```python
from build123d import *

# Parameters (mm, degrees)
BOSS_EXTRUDE1_DEPTH = 2
BOSS_EXTRUDE2_DEPTH = 0.9
SKETCH3_R           = 0.75
CUT_EXTRUDE1_DEPTH  = 0.9
SKETCH4_R           = 0.65
SKETCH4_R_2         = 1.5
CUT_EXTRUDE2_DEPTH  = 0.1
BOSS_EXTRUDE3_DEPTH = 1
SKETCH6_R           = 0.65
BOSS_EXTRUDE4_DEPTH = 5


with BuildPart() as part:
    # Sketch1 → Boss-Extrude1 (new body)
    with BuildSketch(Plane.XY):
        with BuildLine():
            Line((-7.95, 2.1), (7.95, 2.1))
            ThreePointArc((7.95, 2.1), (10.05, 0), (7.95, -2.1))
            Line((7.95, -2.1), (-7.95, -2.1))
            ThreePointArc((-7.95, -2.1), (-10.05, 0), (-7.95, 2.1))
        make_face()
    extrude(amount=BOSS_EXTRUDE1_DEPTH)

    # Sketch2 → Boss-Extrude2 (add)
    with BuildSketch(Plane.XY.offset(2)):
        with BuildLine():
            Line((-10.84, 2.1), (10.84, 2.1))
            ThreePointArc((10.84, 2.1), (12.94, 0), (10.84, -2.1))
            Line((10.84, -2.1), (-10.84, -2.1))
            ThreePointArc((-10.84, -2.1), (-12.94, 0), (-10.84, 2.1))
        make_face()
    extrude(amount=BOSS_EXTRUDE2_DEPTH)

    # Sketch3 → Cut-Extrude1 (cut)
    with BuildSketch(Plane(origin=(0, 0, 2), x_dir=(-1, 0, 0), z_dir=(0, 0, -1))):
        with Locations((-11.49, 0)):
            Circle(SKETCH3_R)
        with Locations((11.49, 0)):
            Circle(SKETCH3_R)
    extrude(amount=-CUT_EXTRUDE1_DEPTH, mode=Mode.SUBTRACT)

    # Sketch4 → Cut-Extrude2 (cut)
    with BuildSketch(Plane(origin=(0, 0, 0), x_dir=(-1, 0, 0), z_dir=(0, 0, -1))):
        Circle(SKETCH4_R)
        with Locations((2.54, 0)):
            Circle(SKETCH4_R)
        with Locations((5.08, 0)):
            Circle(SKETCH4_R)
        with Locations((-2.54, 0)):
            Circle(SKETCH4_R)
        with Locations((-5.08, 0)):
            Circle(SKETCH4_R)
        with Locations((-8, 0)):
            Circle(SKETCH4_R_2)
        with Locations((8, 0)):
            Circle(SKETCH4_R_2)
    extrude(amount=-CUT_EXTRUDE2_DEPTH, mode=Mode.SUBTRACT)

    # Sketch5 → Boss-Extrude3 (add)
    with BuildSketch(Plane.XY.offset(2.9)):
        with BuildLine():
            Line((7.95, 2.1), (-7.95, 2.1))
            ThreePointArc((-7.95, 2.1), (-10.05, 0), (-7.95, -2.1))
            Line((-7.95, -2.1), (7.95, -2.1))
            ThreePointArc((7.95, -2.1), (10.05, 0), (7.95, 2.1))
        make_face()
    extrude(amount=BOSS_EXTRUDE3_DEPTH)

    # Sketch6 → Boss-Extrude4 (add)
    with BuildSketch(Plane.XY.offset(3.9)):
        with Locations(Location((-5.08, 0, 0), (0, 0, 180))):
            Circle(SKETCH6_R)
        with Locations(Location((-2.54, 0, 0), (0, 0, 180))):
            Circle(SKETCH6_R)
        with Locations(Location((0, 0, 0), (0, 0, 180))):
            Circle(SKETCH6_R)
        with Locations(Location((2.54, 0, 0), (0, 0, 180))):
            Circle(SKETCH6_R)
        with Locations(Location((5.08, 0, 0), (0, 0, 180))):
            Circle(SKETCH6_R)
    extrude(amount=BOSS_EXTRUDE4_DEPTH)


solid = part.part
```
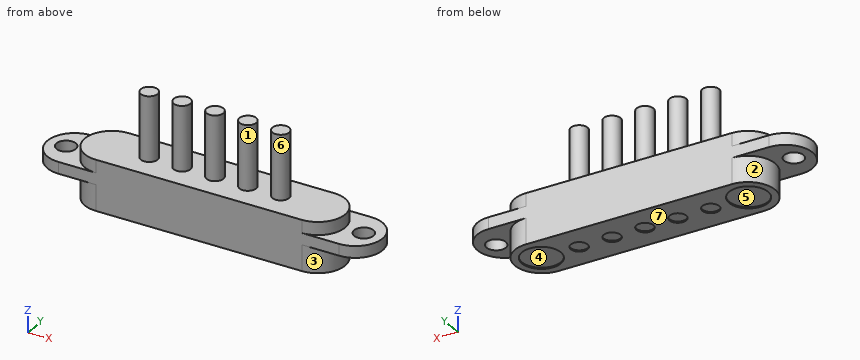
Could you check a few things on this model? Use its own coordinates, in mm. Face numbers are marked on the shaded views. A direction names the side the tool comes from. Give positions to 0.01 mm unless a question says otherwise; leave off trailing zeros. Order: outer loops, then holes, each group sorted by start corner. A loop starts at its lowest first (then second) coordinate and runs counter-clockwise, first axis right, second up.
Q1. Suppose I cut it at A-A, the plane z = 4.5. Write out the boundary of the cut face in (x, y).
Q2. If I drill on line 1 along Y through (x, z) = (8, 0.05); line 2 along Y through (x, z) = (-2.54, 0.05); line 3 along X through (y, z) = (-0.5, 2.75), over which ranges is the centre line in solid material (lowest first)?
Q3. I'm going to push flat-ended pins straight in: P1, Ø1.3, axis at x = -11, y = 0.5, coming from the +Z side; P2, Ø0.8, axis at x = -2.54, y = 0, coming from the -Z side; P3, Ø1.5, axis at y = 1.5, z = 4.5, coming from the +X side. Where does each tip first touch, or does it pass through?
Q4. Suppose I cut it at D-D, the plane y = -1.05. Write out the boundary of the cut face in (x, z).
Q5. Suppose I cut it at C-C, the plane x = -11.49. Write out the boundary of the cut face in (y, z).
Q6. We'd pull the mould along Y, two halves only. Please class the marked faces 5, 6 and 7: +Y half, -Y half, draft (parallel to the pull), parting line (faces both ways), or undercut.
Q7. Suppose I cut it at B-B, the plane x = 0. Write out the boundary of the cut face in (y, z).
Q8. For the marked faces 1, 2, 3 and 4, which set-ups out of +Z, -Z, +X, -X, +Y, -Y let a thin tool reach every point of the face, with its end or its side?
Solution:
1. outline: circle Ø1.3 at (-5.08, 0); circle Ø1.3 at (-2.54, 0); circle Ø1.3 at (0, 0); circle Ø1.3 at (2.54, 0); circle Ø1.3 at (5.08, 0)
2. line 1: y = -2.1 to -1.5, 1.5 to 2.1
2. line 2: y = -2.1 to -0.65, 0.65 to 2.1
2. line 3: x = -12.88 to -12.05, -10.93 to 10.93, 12.05 to 12.88
3. P1: stops at z = 2.9
3. P2: stops at z = 0.1
3. P3: stops at x = 9.77
4. outline: (-12.66, 2) - (-9.77, 2) - (-9.77, 0) - (-9.07, 0) - (-9.07, 0.1) - (-6.93, 0.1) - (-6.93, 0) - (6.93, 0) - (6.93, 0.1) - (9.07, 0.1) - (9.07, 0) - (9.77, 0) - (9.77, 2) - (12.66, 2) - (12.66, 2.9) - (9.77, 2.9) - (9.77, 3.9) - (-9.77, 3.9) - (-9.77, 2.9) - (-12.66, 2.9) - close
5. outline: (-2, 2) - (-0.75, 2) - (-0.75, 2.9) - (-2, 2.9) - close; (0.75, 2) - (2, 2) - (2, 2.9) - (0.75, 2.9) - close
6. face 5: undercut
6. face 6: parting line
6. face 7: draft
7. outline: (-2.1, 0) - (-0.65, 0) - (-0.65, 0.1) - (0.65, 0.1) - (0.65, 0) - (2.1, 0) - (2.1, 3.9) - (0.65, 3.9) - (0.65, 8.9) - (-0.65, 8.9) - (-0.65, 3.9) - (-2.1, 3.9) - close
8. face 1: +Z
8. face 2: -Z, -X
8. face 3: -Z, +X
8. face 4: -Z
